Can you work these out from the model? Positions are in its coordinate system, mm. A direction names the side the tool comes from. Coordinates: 2 decimals unless noted, no trailing zeros. Order: outer loops, then holes, each group sorted by start corner. A loop starts at its lowest first (then second) coordinate and runs counter-clockwise, first axis right, second up. Notation, with made-up numbers: (-33, -35.5) -> (-24, -35.5) arc R26 ccw to (-24, -3.5) -> close; hole circle Ø8 at (27.25, 80). An arc over 180 degrees is marked (long way). Write item = value, one per line.
```python
from build123d import *

# Parameters (mm, degrees)
F1_DEPTH = 100


with BuildPart() as f1:
    # F0 (on Front) → F1 (new body)
    with BuildSketch(Plane.XZ):
        with BuildLine():
            Line((34.869739, -52.836575), (34.869739, 67.163425))
            Line((34.869739, 67.163425), (29.869739, 67.163425))
            ThreePointArc((29.869739, 67.163425), (26.334205, 65.698959), (24.869739, 62.163425))
            Line((24.869739, 62.163425), (24.869739, 52.163425))
            Line((24.869739, 52.163425), (19.869739, 52.163425))
            ThreePointArc((19.869739, 52.163425), (16.334205, 50.698959), (14.869739, 47.163425))
            Line((14.869739, 47.163425), (14.869739, 22.163425))
            ThreePointArc((14.869739, 22.163425), (11.334205, 20.698959), (9.869739, 17.163425))
            Line((9.869739, 17.163425), (9.869739, -12.836575))
            ThreePointArc((9.869739, -12.836575), (6.334205, -14.301041), (4.869739, -17.836575))
            Line((4.869739, -17.836575), (4.869739, -52.836575))
            Line((4.869739, -52.836575), (34.869739, -52.836575))
        make_face()
    extrude(amount=F1_DEPTH)


solid = f1.part
```
Item 1: I want a section at C-C, the plane x = 23. Please give me the cut outline in (y, z).
A:
outline = (-100, -52.84) -> (0, -52.84) -> (0, 52.16) -> (-100, 52.16) -> close
Item 2: For faces 1 (the flat face through (23, 0, -5)), 2 (the flat face through (14.87, -49, 35)), which set-ups out of +Z, -Z, +X, -X, +Y, -Y let a thin tool reach every point of the face, with its end or its side?
A:
face_1 = +Z, -Z, +X, -X, +Y
face_2 = +Z, -X, +Y, -Y
Item 3: If I drill on probe 1 along X at (y, z) = (-68, 7.5); probe 2 along Z at (x, y) = (20, -60); probe 3 along X at (y, z) = (-23, 46.5), over which ranges is the centre line in solid material (lowest first)?
A:
probe_1 = 9.87 to 34.87
probe_2 = -52.84 to 52.16
probe_3 = 14.87 to 34.87
Item 4: I'm going to push flat-ended pins straight in: P1, Ø12.5, axis at y = -70.5, z = 31.5, coming from the -X side; P2, Ø24, axis at y = -60, z = 0.5, coming from the -X side; P3, Ø1, axis at x = 14, y = -14, coming from the +Z side; P4, Ø5, axis at x = 11.5, z = 24.5, coming from the +Y side. Where does each tip first touch, or does it pass through?
A:
P1 = 14.87
P2 = 9.87
P3 = 22.15
P4 = through
Item 5: I want a section at B-B, the plane z = 29. Please give me the cut outline in (x, y).
A:
outline = (14.87, -100) -> (34.87, -100) -> (34.87, 0) -> (14.87, 0) -> close
Item 6: I want a section at A-A, the plane y = -11.5. Please give me the cut outline in (x, z).
A:
outline = (4.87, -52.84) -> (34.87, -52.84) -> (34.87, 67.16) -> (29.87, 67.16) arc R5 ccw to (24.87, 62.16) -> (24.87, 52.16) -> (19.87, 52.16) arc R5 ccw to (14.87, 47.16) -> (14.87, 22.16) arc R5 ccw to (9.87, 17.16) -> (9.87, -12.84) arc R5 ccw to (4.87, -17.84) -> close
